from build123d import *

# Parameters (mm, degrees)
BOSS_EXTRUDE1_DEPTH = 7
SKETCH3_R           = 37.663730654
CUT_EXTRUDE1_DEPTH  = 88.594763353
CIRPATTERN1_COUNT   = 8
SKETCH8_W           = 10
SKETCH8_H           = 10
BOSS_EXTRUDE2_DEPTH = 95
SKETCH9_W           = 10
SKETCH9_H           = 10
SKETCH9_R           = 2.5
CUT_EXTRUDE2_DEPTH  = 5
CUT_EXTRUDE3_DEPTH  = 135.267801676
SKETCH11_R          = 2.5
CUT_EXTRUDE4_DEPTH  = 135.267801676
CIRPATTERN2_COUNT   = 4
FILLET1_R           = 2


with BuildPart() as part:
    # Sketch1 → Boss-Extrude1 (new body)
    with BuildSketch(Plane(origin=(0, 0, 0), x_dir=(1, 0, 0), z_dir=(0, 1, 0))):
        with BuildLine():
            Line((-8, 56.940758688), (-8, 59.740758688))
            ThreePointArc((-8, 59.740758688), (-7.414213562, 61.154972251), (-6, 61.740758688))
            Line((-6, 61.740758688), (6, 61.740758688))
            ThreePointArc((6, 61.740758688), (7.414213562, 61.154972251), (8, 59.740758688))
            Line((8, 59.740758688), (8, 56.940758688))
            ThreePointArc((8, 56.940758688), (22.004297361, 53.123073119), (34.606342345, 45.920050844))
            Line((34.606342345, 45.920050844), (36.586241332, 47.899949831))
            ThreePointArc((36.586241332, 47.899949831), (38.000454895, 48.485736269), (39.414668457, 47.899949831))
            Line((39.414668457, 47.899949831), (47.899949831, 39.414668457))
            ThreePointArc((47.899949831, 39.414668457), (48.485736269, 38.000454895), (47.899949831, 36.586241332))
            Line((47.899949831, 36.586241332), (45.920050844, 34.606342345))
            ThreePointArc((45.920050844, 34.606342345), (53.123073119, 22.004297361), (56.940758688, 8))
            Line((56.940758688, 8), (59.740758688, 8))
            ThreePointArc((59.740758688, 8), (61.154972251, 7.414213562), (61.740758688, 6))
            Line((61.740758688, 6), (61.740758688, -6))
            ThreePointArc((61.740758688, -6), (61.154972251, -7.414213562), (59.740758688, -8))
            Line((59.740758688, -8), (56.940758688, -8))
            ThreePointArc((56.940758688, -8), (53.123073119, -22.004297361), (45.920050844, -34.606342345))
            Line((45.920050844, -34.606342345), (47.899949831, -36.586241332))
            ThreePointArc((47.899949831, -36.586241332), (48.485736269, -38.000454895), (47.899949831, -39.414668457))
            Line((47.899949831, -39.414668457), (39.414668457, -47.899949831))
            ThreePointArc((39.414668457, -47.899949831), (38.000454895, -48.485736269), (36.586241332, -47.899949831))
            Line((36.586241332, -47.899949831), (34.606342345, -45.920050844))
            ThreePointArc((34.606342345, -45.920050844), (22.004297361, -53.123073119), (8, -56.940758688))
            Line((8, -56.940758688), (8, -59.740758688))
            ThreePointArc((8, -59.740758688), (7.414213562, -61.154972251), (6, -61.740758688))
            Line((6, -61.740758688), (-6, -61.740758688))
            ThreePointArc((-6, -61.740758688), (-7.414213562, -61.154972251), (-8, -59.740758688))
            Line((-8, -59.740758688), (-8, -56.940758688))
            ThreePointArc((-8, -56.940758688), (-22.004297361, -53.123073119), (-34.606342345, -45.920050844))
            Line((-34.606342345, -45.920050844), (-36.586241332, -47.899949831))
            ThreePointArc((-36.586241332, -47.899949831), (-38.000454895, -48.485736269), (-39.414668457, -47.899949831))
            Line((-39.414668457, -47.899949831), (-47.899949831, -39.414668457))
            ThreePointArc((-47.899949831, -39.414668457), (-48.485736269, -38.000454895), (-47.899949831, -36.586241332))
            Line((-47.899949831, -36.586241332), (-45.920050844, -34.606342345))
            ThreePointArc((-45.920050844, -34.606342345), (-53.123073119, -22.004297361), (-56.940758688, -8))
            Line((-56.940758688, -8), (-59.740758688, -8))
            ThreePointArc((-59.740758688, -8), (-61.154972251, -7.414213562), (-61.740758688, -6))
            Line((-61.740758688, -6), (-61.740758688, 6))
            ThreePointArc((-61.740758688, 6), (-61.154972251, 7.414213562), (-59.740758688, 8))
            Line((-59.740758688, 8), (-56.940758688, 8))
            ThreePointArc((-56.940758688, 8), (-53.123073119, 22.004297361), (-45.920050844, 34.606342345))
            Line((-45.920050844, 34.606342345), (-47.899949831, 36.586241332))
            ThreePointArc((-47.899949831, 36.586241332), (-48.485736269, 38.000454895), (-47.899949831, 39.414668457))
            Line((-47.899949831, 39.414668457), (-39.414668457, 47.899949831))
            ThreePointArc((-39.414668457, 47.899949831), (-38.000454895, 48.485736269), (-36.586241332, 47.899949831))
            Line((-36.586241332, 47.899949831), (-34.606342345, 45.920050844))
            ThreePointArc((-34.606342345, 45.920050844), (-22.004297361, 53.123073119), (-8, 56.940758688))
        make_face()
    extrude(amount=BOSS_EXTRUDE1_DEPTH)

    # Sketch3 → Cut-Extrude1 (cut, through all)
    with BuildSketch(Plane(origin=(0, 7, 0), x_dir=(1, 0, 0), z_dir=(0, 1, 0))):
        with Locations(Location((0, 0, 0), (0, 0, 270))):
            Circle(SKETCH3_R)
    extrude(amount=-CUT_EXTRUDE1_DEPTH, mode=Mode.SUBTRACT)

    # Sketch7 → Cut-Loft1 section 0
    with BuildSketch(Plane.XZ):
        with BuildLine():
            Line((-6, -57.040758688), (6, -57.040758688))
            Line((6, -57.040758688), (6, -59.340758688))
            Line((6, -59.340758688), (-6, -59.340758688))
            Line((-6, -59.340758688), (-6, -57.040758688))
        make_face()
    # Sketch5 → Cut-Loft1 section 1
    with BuildSketch(Plane(origin=(0, 7, 0), x_dir=(1, 0, 0), z_dir=(0, 1, 0))):
        with BuildLine():
            Line((-6, 59.740758688), (6, 59.740758688))
            Line((6, 59.740758688), (6, 57.040758688))
            Line((6, 57.040758688), (-6, 57.040758688))
            Line((-6, 57.040758688), (-6, 59.740758688))
        make_face()
    cut_loft1 = loft(mode=Mode.SUBTRACT)

    # CirPattern1: Cut-Loft1 ×8 about axis
    cirpattern1_axis = Axis((0, 0, 0), (0, 1, 0))
    for i in range(1, CIRPATTERN1_COUNT):
        add(cut_loft1.rotate(cirpattern1_axis, i * 360 / CIRPATTERN1_COUNT), mode=Mode.SUBTRACT)

    # Sketch8 → Boss-Extrude2 (add)
    with BuildSketch(Plane(origin=(0, 7, 0), x_dir=(1, 0, 0), z_dir=(0, 1, 0))):
        with Locations((45, 5)):
            Rectangle(SKETCH8_W, SKETCH8_H)
        with Locations((-45, 5)):
            Rectangle(SKETCH8_W, SKETCH8_H)
    extrude(amount=BOSS_EXTRUDE2_DEPTH)

    # Sketch9 → Cut-Extrude2 (cut)
    with BuildSketch(Plane.XY):
        with Locations((-45, 97)):
            Rectangle(SKETCH9_W, SKETCH9_H)
        with Locations((-45, 97)):
            Circle(SKETCH9_R, mode=Mode.SUBTRACT)
    cut_extrude2 = extrude(amount=-CUT_EXTRUDE2_DEPTH, mode=Mode.SUBTRACT)

    # Sketch9<2> → Cut-Extrude3 (cut, through all)
    with BuildSketch(Plane.XY):
        with BuildLine():
            ThreePointArc((-42.5, 97), (-42.690301169, 97.956708581), (-43.232233047, 98.767766953))
            Line((-43.232233047, 98.767766953), (-46.767766953, 95.232233047))
            ThreePointArc((-46.767766953, 95.232233047), (-44.043291419, 94.690301169), (-42.5, 97))
        make_face()
        with BuildLine():
            Line((-46.767766953, 95.232233047), (-43.232233047, 98.767766953))
            ThreePointArc((-43.232233047, 98.767766953), (-46.767766953, 98.767766953), (-46.767766953, 95.232233047))
        make_face()
    cut_extrude3 = extrude(amount=-CUT_EXTRUDE3_DEPTH, mode=Mode.SUBTRACT)

    # Mirror1: Cut-Extrude2, Cut-Extrude3 across plane
    add(cut_extrude2.mirror(Plane(origin=(0, 0, 0), x_dir=(0, 0, 1), z_dir=(1, 0, 0))), mode=Mode.SUBTRACT)
    add(cut_extrude3.mirror(Plane(origin=(0, 0, 0), x_dir=(0, 0, 1), z_dir=(1, 0, 0))), mode=Mode.SUBTRACT)

    # Sketch11 → Cut-Extrude4 (cut, through all)
    with BuildSketch(Plane.XZ):
        with Locations(Location((-31.819805153, -31.819805153, 0), (0, 0, 270))):
            Circle(SKETCH11_R)
    cut_extrude4 = extrude(amount=-CUT_EXTRUDE4_DEPTH, mode=Mode.SUBTRACT)

    # CirPattern2: Cut-Extrude4 ×4 about axis
    cirpattern2_axis = Axis((0, 0, 0), (0, 1, 0))
    for i in range(1, CIRPATTERN2_COUNT):
        add(cut_extrude4.rotate(cirpattern2_axis, i * 360 / CIRPATTERN2_COUNT), mode=Mode.SUBTRACT)

    # Fillet1
    fillet1_edges = [part.edges().sort_by_distance(p)[0] for p in [
        (50, 7, -5),
        (45, 7, -10),
        (40, 7, -5),
        (45, 7, 0),
        (-45, 7, -10),
        (-50, 7, -5),
        (-45, 7, 0),
        (-40, 7, -5),
    ]]
    fillet(fillet1_edges, radius=FILLET1_R)


solid = part.part
The model under review builds one solid part; all positions refer to its coordinate system, in mm. A direction names the side the tool comes from. Round coordinates to 2 decimals unless told otherwise and drop trailing zeros. Write each loop counter-clockwise with the first axis right and the second up, starting at its lowest first coordinate (ties: lowest second). Pieces come first, ordered by that corner, then holes. Notation, with made-up numbers: (32.25, -24) -> (67.25, -24) arc R30 ccw to (67.25, 3) -> close; hole circle Ø2 at (-32.75, -19.75). An arc over 180 degrees is marked (long way). Answer as a JSON object with one key per item and string values.
1. We need section C-C on z = -21. State the section outline as (x, y) points, and give its area (3 significant figures).
Results found:
{"outline": "(-53.53, 0) -> (-31.27, 0) -> (-31.27, 7) -> (-53.53, 7) -> close; (31.27, 0) -> (53.53, 0) -> (53.53, 7) -> (31.27, 7) -> close", "area": "312 mm^2"}
2. To check wall thickness, follow line 1 along Y through (x, z) = (-11.5, -48); line 2 along X through (y, z) = (22, -7); line 3 along Z through (x, y) = (-49, 35). State the ranges of each line that lie inside material, in increasing order.
Results found:
{"line 1": "y = 0 to 7", "line 2": "x = -50 to -40, 40 to 50", "line 3": "z = -10 to 0"}
3. Clearance check with flat-ended pins moving along their axes: pin 1 (1.4 mm diameter, centred on y = 4.5, z = 58, fed in from -X); pin 2 (1.5 mm diameter, centred on x = -46.5, z = -2, fed in from +Y); pin 3 (11 mm diameter, centred on y = 59, z = -6, fed in from +X); pin 4 (4.5 mm diameter, centred on x = 31.82, z = 31.82, fed in from -Y) (1 decimal). State where each tip first meets the part, or that it passes through.
Results found:
{"pin 1": "stops at x = -8", "pin 2": "stops at y = 92", "pin 3": "stops at x = 50", "pin 4": "passes through"}
4. We need section B-B on y = 37.5. State the section outline as (x, z) points.
Results found:
{"outline": "(-50, -10) -> (-40, -10) -> (-40, 0) -> (-50, 0) -> close; (40, -10) -> (50, -10) -> (50, 0) -> (40, 0) -> close"}
5. Machinability: for faces 4 (the face through (0, 3, 61.741)), 5 (the face through (42.044, 3.549, 42.163)), 6 (the face through (47, 99, -5)), 7 (the face through (61.741, 3, 0)), 8 (the face through (-40.393, 3.549, -40.275)), which of the approach directions +Z, -Z, +X, -X, +Y, -Y give a long, thin tool a straight path to every point of the face, cutting with its end or side? Answer none if there is none.
Results found:
{"face 4": "+Z, +X, -X, +Y, -Y", "face 5": "+Y", "face 6": "+Z, +X, -X, +Y", "face 7": "+Z, -Z, +X, +Y, -Y", "face 8": "+Y, -Y"}
6. The part is to be moulded in two halves that separate along X. For faces 1 (the face through (-45, 50, 0)), 2 (the face through (53.2, 3.45, 21.82)), 3 (the face through (-29.322, 3.451, 31.71)), say which applies: pulls with the +X half, pulls with the -X half, needs draft (parallel to the pull), parting line crosses it, or undercut.
Results found:
{"face 1": "needs draft", "face 2": "pulls with the +X half", "face 3": "undercut"}
7. We need section A-A on x = 0. State the section outline as (y, z) points, and give its area (3 significant figures).
Results found:
{"outline": "(0, -61.74) -> (7, -61.74) -> (7, -59.74) -> (0, -59.34) -> close; (0, -57.04) -> (7, -57.04) -> (7, -37.66) -> (0, -37.66) -> close; (0, 37.66) -> (7, 37.66) -> (7, 57.04) -> (0, 57.04) -> close; (0, 59.34) -> (7, 59.74) -> (7, 61.74) -> (0, 61.74) -> close", "area": "302 mm^2"}
